```python
from build123d import *

# Parameters (mm, degrees)
SKETCH_2_W             = 260
SKETCH_2_H             = 117.5
EXTRUDE_1_DEPTH        = 20
CUT_EXTRUDE_1_DEPTH    = 287.017919019
PATTERN_LINEAR_1_COUNT = 3
PATTERN_LINEAR_1_PITCH = 100
SKETCH_4_W             = 200
SKETCH_4_H             = 30
EXTRUDE_2_DEPTH        = 100
SKETCH_5_R             = 30
CUT_EXTRUDE_2_DEPTH    = 300.42653523


with BuildPart() as part:
    # 草图2 → 凸台-拉伸1 (new body)
    with BuildSketch(Plane(origin=(0, 0, 0), x_dir=(1, 0, 0), z_dir=(0, 1, 0))):
        with Locations((130, -58.75)):
            Rectangle(SKETCH_2_W, SKETCH_2_H)
    extrude(amount=EXTRUDE_1_DEPTH)

    # 草图3 → 切除-拉伸1 (cut, through all)
    with BuildSketch(Plane(origin=(0, 20, 0), x_dir=(1, 0, 0), z_dir=(0, 1, 0))):
        with BuildLine():
            Line((20, -58.5), (40, -58.5))
            ThreePointArc((40, -58.5), (49, -67.5), (40, -76.5))
            Line((40, -76.5), (20, -76.5))
            ThreePointArc((20, -76.5), (11, -67.5), (20, -58.5))
        make_face()
    cut_extrude_1 = extrude(amount=-CUT_EXTRUDE_1_DEPTH, mode=Mode.SUBTRACT)

    # 阵列(线性)1: 切除-拉伸1 ×3
    with Locations(*[(i * PATTERN_LINEAR_1_PITCH, 0, 0) for i in range(1, PATTERN_LINEAR_1_COUNT)]):
        add(cut_extrude_1, mode=Mode.SUBTRACT)

    # 草图4 → 凸台-拉伸2 (add)
    with BuildSketch(Plane(origin=(0, 20, 0), x_dir=(1, 0, 0), z_dir=(0, 1, 0))):
        with Locations((130, -15)):
            Rectangle(SKETCH_4_W, SKETCH_4_H)
    extrude(amount=EXTRUDE_2_DEPTH)

    # 草图5 → 切除-拉伸2 (cut, through all)
    with BuildSketch(Plane.XY.offset(30)):
        with Locations((130, 70)):
            Circle(SKETCH_5_R)
        with BuildLine():
            Line((30, 70), (105, 113.301270189))
            ThreePointArc((105, 113.301270189), (130, 120), (155, 113.301270189))
            Line((155, 113.301270189), (230, 70))
            Line((230, 70), (230, 137.29910678))
            Line((230, 137.29910678), (30, 137.29910678))
            Line((30, 137.29910678), (30, 70))
        make_face()
    extrude(amount=-CUT_EXTRUDE_2_DEPTH, mode=Mode.SUBTRACT)


solid = part.part
```
Can you work these out from the model? Positions are in its coordinate system, mm. A direction names the side the tool comes from. Give positions to 0.01 mm unless a question says otherwise; leave off trailing zeros. Order: outer loops, then holes, each group sorted by start corner. A loop starts at its lowest first (then second) coordinate and runs counter-clockwise, first axis right, second up. Notation, with made-up numbers: M 35,9.25 L 83,9.25 A28 ccw 83,28.25 Z; hole C 56,-34.5 d10. An arc over 180 degrees is marked long. Write item = value, one per line. Start each with the question number.
Q1. Suppose I cut it at D-D (x = 37.5). Write out the boundary of the cut face in (y, z).
Q2. I need wall thicknesses on probe 1 along Y at (x, z) = (130, 15.5); probe 2 along Z at (x, y) = (96, 51); probe 3 along Y at (x, z) = (225.5, 91). Which ranges of each line are inside material? Lowest first, please. Write a range as [from, to].
Q3. Suppose I cut it at B-B (x = 130). Write out the boundary of the cut face in (y, z).
Q4. Suppose I cut it at C-C (y = 59). Write out the boundary of the cut face in (x, z), plus the area to 3 significant figures.
Q5. We'd pull the mould along X, two halves only. Please class faces 1 (the flat face through (30, 10, 76.5)), 2 (the flat face through (128, 32, 0)), 3 (the flat face through (66.98, 91.35, 15.21)): pulls with the +X half, pulls with the -X half, needs draft (parallel to the pull), parting line crosses it, or undercut.
Q6. Suppose I cut it at A-A (z = 67.5). Write out the boundary of the cut face in (x, y), plus the area to 3 significant figures.
Q7. For faces 4 (the flat face through (30, 10, 58.5)), 5 (the flat face through (129, 36, 30)), 6 (the flat face through (230, 45, 15)), 7 (the cylindrical face through (130, 120, 15)), which set-ups out of +Z, -Z, +X, -X, +Y, -Y let a thin tool reach every point of the face, with its end or its side?
Q8. Will these pins go through, and if not, where does the flat tip stop? pin 1 Ø1 at (y, z) = (23, 16) entering from -X; pin 2 Ø15 at (y, z) = (44, 13) entering from +X; pin 3 Ø10 at (x, z) = (146.5, 58.5) entering from +Y.
Check result:
q1.outline = M 0,0 L 74.33,0 L 74.33,30 L 20,30 L 20,58.5 L 0,58.5 Z; M 0,76.5 L 20,76.5 L 20,117.5 L 0,117.5 Z
q2.probe_1 = [0, 40], [100, 120]
q2.probe_2 = [0, 30]
q2.probe_3 = [0, 20]
q3.outline = M 0,0 L 40,0 L 40,30 L 20,30 L 20,58.5 L 0,58.5 Z; M 0,76.5 L 20,76.5 L 20,117.5 L 0,117.5 Z; M 100,0 L 120,0 L 120,30 L 100,30 Z
q4.outline = M 30,0 L 102.09,0 L 102.09,30 L 30,30 Z; M 157.91,0 L 230,0 L 230,30 L 157.91,30 Z
q4.area = 4,330 mm2
q5.face_1 = undercut
q5.face_2 = needs draft
q5.face_3 = pulls with the -X half
q6.outline = M 0,0 L 11,0 L 11,20 L 0,20 Z; M 49,0 L 111,0 L 111,20 L 49,20 Z; M 149,0 L 211,0 L 211,20 L 149,20 Z; M 249,0 L 260,0 L 260,20 L 249,20 Z
q6.area = 2,920 mm2
q7.face_4 = +Y, -Y
q7.face_5 = +Z, +X, -X, +Y
q7.face_6 = +Z, -Z, +X, +Y
q7.face_7 = +Z, -Z, +Y
q8.pin_1 = 30
q8.pin_2 = 230
q8.pin_3 = 20
